Read the model definition and answer for the solid it produces. Units are mm, in the model's axes. Face numbers are marked on the shaded views. A direction names the side the tool comes from. Give positions to 0.01 mm unless a question says otherwise; leave off trailing zeros. Loops run counter-clockwise (first coordinate to the right, second up) from the corner with the lowest first, then second, coordinate; pieces in that order, holes last. Notation, with made-up numbers: M 78.5,65 L 91.5,65 A22 ccw 91.5,71 Z; hole C 19.5,-7.75 d3. An arc over 180 degrees is marked long. Return JSON: item names as keys, results as strings. Group by question number.
```python
from build123d import *

# Parameters (mm, degrees)
F0_W     = 203.2
F0_H     = 111.76
F1_DEPTH = 12.7
F2_W     = 12.7
F2_H     = 101.6
F3_DEPTH = 152.4
F5_D     = 25.4
F6_R     = 50.79999
F7_R     = 50.79999
F8_W     = 50.8
F8_H     = 12.7
F9_DEPTH = 50.8
F10_SIZE = 50.79999


# Not quite as in the source:
# - a fillet or chamfer is up to 0.001 mm smaller than in the source, because OpenCascade refuses the exact size
# - a feature names something its author has since deleted; it is built from what else it names


with BuildPart() as f1:
    # F0 (on Top) → F1 (new body)
    with BuildSketch(Plane.XY):
        with Locations((0, -2.54)):
            Rectangle(F0_W, F0_H)
    extrude(amount=F1_DEPTH)

    # F2 (on face) → F3 (join)
    with BuildSketch(Plane.XY.offset(12.7)):
        with Locations((-88.9, -2.54)):
            Rectangle(F2_W, F2_H)
        with Locations((88.9, -2.54)):
            Rectangle(F2_W, F2_H)
    extrude(amount=F3_DEPTH)

    # F5 (through all)
    with Locations(Plane.YZ.offset(95.25)):
        with Locations((0, 140.1294022799)):
            Hole(F5_D / 2)

    # F6 (radius 50.8 in the source; OpenCascade refuses exactly that, so slightly less here)
    f6_edges = [f1.edges().sort_by_distance(p)[0] for p in [
        (-88.9, -53.34, 165.1),
        (-88.9, 48.26, 165.1),
    ]]
    fillet(f6_edges, radius=F6_R)

    # F7 (radius 50.8 in the source; OpenCascade refuses exactly that, so slightly less here)
    f7_edges = [f1.edges().sort_by_distance(p)[0] for p in [
        (88.9, -53.34, 165.1),
        (88.9, 48.26, 165.1),
    ]]
    fillet(f7_edges, radius=F7_R)

    # F8 (on face) → F9 (join)
    with BuildSketch(Plane.XY.offset(12.7)):
        with Locations((-57.15, -2.54)):
            Rectangle(F8_W, F8_H)
        with Locations((57.15, -2.54)):
            Rectangle(F8_W, F8_H)
    extrude(amount=F9_DEPTH)

    # F10 (size 50.8 in the source; OpenCascade refuses exactly that, so slightly less here)
    f10_edges = [f1.edges().sort_by_distance(p)[0] for p in [
        (-31.75, -2.54, 63.5),
        (31.75, -2.54, 63.5),
    ]]
    chamfer(f10_edges, length=F10_SIZE)


solid = f1.part
```
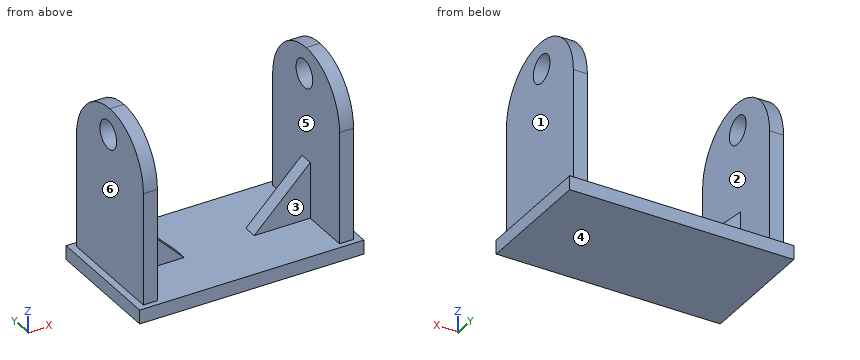
1. Flat-ended cylindrical pins translate along their axes: P1, Ø4, axis at y = 26.5, z = 32.5, coming from the -X side; P2, Ø4, axis at x = -89.5, z = 80, coming from the -Y side; P3, Ø1.5, axis at y = 21, z = 127.5, coming from the +X side. Find the tip coordinate at first contact, or state that the pin passes through.
2. Find section D-D (y = -23.5). Write down the section's boundary in (x, z), and give its area (3 significant figures).
3. Find section C-C (x = -39.5). Write down the section's boundary in (y, z).
4. Find section A-A (z = 50). Write down the section's boundary in (x, y), and give its area (3 significant figures).
5. Find section B-B (y = 0). State how many separate pieces and enclosed holes the cut face has, and give its area (3 significant figures).
6. The mould has two halves that part along X. Classify the marked faces 4, 5 and 6: +X half, -X half, draft (parallel to the pull), parting line (faces both ways), or undercut.
7. For the marked faces 1, 2 and 3, determine the directions among +Z, -Z, +X, -X, +Y, -Y from which every point of the face is accessible in a straight line to the end or side of a thin tool.
8. Straight lines are drawn through the part: line 1 along X through (y, z) = (34, 90); line 2 along Z through (x, y) = (-17.5, 41); line 3 along Z through (x, y) = (-87.5, 6.5). For each, find the intervals that lie inside material, in ascending order.
Result:
{
 "1": {"P1": "stops at x = -95.25", "P2": "stops at y = -53.34", "P3": "stops at x = 95.25"},
 "2": {"outline": "M -101.6,0 L 101.6,0 L 101.6,12.7 L 95.25,12.7 L 95.25,160.57 L 82.55,160.57 L 82.55,12.7 L -82.55,12.7 L -82.55,160.57 L -95.25,160.57 L -95.25,12.7 L -101.6,12.7 Z", "area": "6,340 mm2"},
 "3": {"outline": "M -58.42,0 L 53.34,0 L 53.34,12.7 L 3.81,12.7 L 3.81,20.45 L -8.89,20.45 L -8.89,12.7 L -58.42,12.7 Z"},
 "4": {"outline": "M -95.25,-53.34 L -82.55,-53.34 L -82.55,-8.89 L -69.05,-8.89 L -69.05,3.81 L -82.55,3.81 L -82.55,48.26 L -95.25,48.26 Z; M 69.05,-8.89 L 82.55,-8.89 L 82.55,-53.34 L 95.25,-53.34 L 95.25,48.26 L 82.55,48.26 L 82.55,3.81 L 69.05,3.81 Z", "area": "2,920 mm2"},
 "5": {"separate pieces": "3", "enclosed holes": "0", "area": "8,390 mm2"},
 "6": {"face 4": "draft", "face 5": "undercut", "face 6": "-X half"},
 "7": {"face 1": "+Z, +X, +Y, -Y", "face 2": "+Z", "face 3": "+Z, -Y"},
 "8": {"line 1": "x = -95.25 to -82.55, 82.55 to 95.25", "line 2": "z = 0 to 12.7", "line 3": "z = 0 to 129.22, 151.04 to 164.29"}
}
